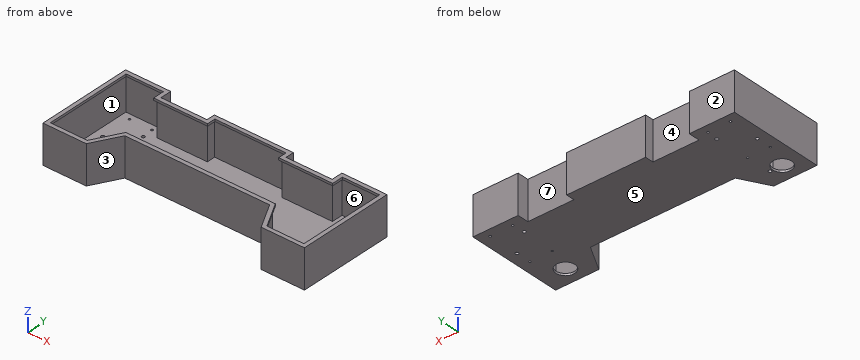
```python
from build123d import *

# Parameters (mm, degrees)
EXTRUDE_1_DEPTH         = 20.5
SCALE_1_SCALE           = 10
SHELL_1_T               = -11
EXTRUDE_2_DEPTH         = 12
HOLE_WIZARD_17_0_17_1_D = 17
M12X1_25_2_D            = 10.5
F_12_0MM_1_D            = 12
SKETCH_27_R             = 50
CUT_EXTRUDE_1_DEPTH     = 11


with BuildPart() as part:
    # 草图1 → 凸台-拉伸1 (new body)
    with BuildSketch(Plane.XY):
        Polygon((-61.070262854, 36.5), (-37.070262854, 36.5), (-37.070262854, 30.5), (-12.570262854, 30.5), (-12.570262854, 35), (29.429737146, 35), (29.429737146, 30.5), (53.929737146, 30.5), (53.929737146, 36.5), (77.929737146, 36.5), (77.929737146, -14.5), (54.929737146, -14.5), (46.929737146, 0), (-30.070262854, 0), (-38.070262854, -14.5), (-61.070262854, -14.5), align=None)
    extrude(amount=EXTRUDE_1_DEPTH)


with BuildPart() as part_1:
    # 缩放比例1: scaled about (8.429737146, 13.654642846, 10.25)
    add(part.part.scale(SCALE_1_SCALE).moved(Location((-75.867634314, -122.891785614, -92.25))))

    # 抽壳1
    shell_1_openings = [part_1.faces().sort_by_distance(p)[0] for p in [
        (8.429737147, 13.654642849, 112.75),
    ]]
    offset(amount=SHELL_1_T, openings=shell_1_openings, kind=Kind.INTERSECTION)

    # 草图12 → 凸台-拉伸2 (add)
    with BuildSketch(Plane.XY.offset(112.75)):
        Polygon((-675.570262854, 231.108214383), (-675.570262854, -256.891785617), (-463.064431597, -256.891785617), (-383.064431597, -111.891785617), (399.923905889, -111.891785617), (479.923905889, -256.891785617), (692.429737146, -256.891785617), (692.429737146, 231.108214383), (474.429737146, 231.108214383), (474.429737146, 171.108214383), (207.429737146, 171.108214383), (207.429737146, 216.108214383), (-190.570262854, 216.108214383), (-190.570262854, 171.108214383), (-457.570262854, 171.108214383), (-457.570262854, 231.108214383), align=None)
        Polygon((-665.570262854, 221.108214383), (-665.570262854, -246.891785617), (-468.968221364, -246.891785617), (-388.968221364, -101.891785617), (405.827695656, -101.891785617), (485.827695656, -246.891785617), (682.429737146, -246.891785617), (682.429737146, 221.108214383), (484.429737146, 221.108214383), (484.429737146, 161.108214383), (197.429737146, 161.108214383), (197.429737146, 206.108214383), (-180.570262854, 206.108214383), (-180.570262854, 161.108214383), (-467.570262854, 161.108214383), (-467.570262854, 221.108214383), align=None, mode=Mode.SUBTRACT)
    extrude(amount=-EXTRUDE_2_DEPTH)

    # Ø17.0 (17) 直径孔1 (through all)
    with Locations(Plane.XY.offset(-81.25)):
        with Locations((-505.570262854, 141.108214383), (-630.570262854, 36.108214383), (-515.570262854, -176.891785617), (647.429737146, 36.108214383), (522.429737146, 136.108214383), (532.429737146, -176.891785617)):
            Hole(HOLE_WIZARD_17_0_17_1_D / 2)

    # M12x1.25 螺纹孔2 (through all)
    with Locations(Plane.XY.offset(-81.25)):
        with Locations((-630.570262854, -43.891785617), (-510.570262854, -43.891785617), (527.429737146, -43.891785617), (647.429737146, -43.891785617)):
            Hole(M12X1_25_2_D / 2)

    # Ø12.0mm 暗销孔1 (through all)
    with Locations(Plane(origin=(-630.570262854, 201.108214383, -81.25), x_dir=(1, 0, 0), z_dir=(0, 0, 1))):
        with Locations((0, 0), (120, 0), (1158, 0), (1278, 0)):
            Hole(F_12_0MM_1_D / 2)

    # 草图27 → 切除-拉伸1 (cut)
    with BuildSketch(Plane.XY.offset(-81.25)):
        with Locations((572.429737146, -176.891785617)):
            Circle(SKETCH_27_R)
        with Locations((-579.570262855, -176.891785617)):
            Circle(SKETCH_27_R)
    extrude(amount=-CUT_EXTRUDE_1_DEPTH, mode=Mode.SUBTRACT)


solid = part_1.part
```
Source: CAD feature listing. Evaluate the final solid. Frame: model axes, mm. Face numbers are marked on the shaded views. A direction names the side the tool comes from. Coordinates: 2 decimals unless noted, no trailing zeros. Write each loop counter-clockwise with the first axis right and the second up, starting at its lowest first coordinate (ties: lowest second). Pieces come first, ordered by that corner, then holes. Notation, with made-up numbers: (64, 26) -> (113, 26) arc R28 ccw to (113, 51) -> close; hole circle Ø6 at (-29.75, 36). An arc over 180 degrees is marked (long way). Return JSON: item names as keys, results as strings. Group by question number.
1) Section query C-C, the plane y = -66. Return loops of the section in (x, z).
2) Section query B-B, the plane x = -292. Return loops of the section in (y, z), plus the area to 3 significant figures.
3) Mould query, pull axis Z, two halves, no side actions, for the marked faces 5, 6 and 7. Classes: +Z half, -Z half, draft (parallel to the pull), parting line (faces both ways), or undercut.
4) Set-up query: the marked faces 1, 2, 3 and 4. Return all of +Z, -Z, +X, -X, +Y, -Y with unobstructed straight access to the full face (end or side cutting, diameter ignored); none if empty.
5) Ray query, line 1 along X through (y, z) = (186, 27.5); line 2 along X through (y, z) = (27, 56.5); line 3 along Y through (x, z) = (197.5, 95.5). Return the intervals inside material, ascending.
6) Contact query for flat-ended pins moving along their axis: P1, Ø2, axis at x = -332, z = 69.5, coming from the +Y side; P2, Ø12, axis at x = 647.43, y = -43.89, coming from the +Z side; P3, Ø1, axis at x = -221.5, z = 73, coming from the -Y side. Output: stop coordinate, or through.
From the geometry:
{
 "1": {"outline": "(-686.57, -92.25) -> (703.43, -92.25) -> (703.43, 112.75) -> (682.43, 112.75) -> (682.43, 100.75) -> (692.43, 100.75) -> (692.43, -81.25) -> (-675.57, -81.25) -> (-675.57, 100.75) -> (-665.57, 100.75) -> (-665.57, 112.75) -> (-686.57, 112.75) -> close"},
 "2": {"outline": "(-122.89, -92.25) -> (182.11, -92.25) -> (182.11, 112.75) -> (161.11, 112.75) -> (161.11, 100.75) -> (171.11, 100.75) -> (171.11, -81.25) -> (-111.89, -81.25) -> (-111.89, 100.75) -> (-101.89, 100.75) -> (-101.89, 112.75) -> (-122.89, 112.75) -> close", "area": "7,860 mm²"},
 "3": {"face 5": "-Z half", "face 6": "undercut", "face 7": "draft"},
 "4": {"face 1": "none", "face 2": "+Z, -Z, +X, -X, +Y", "face 3": "+Z, -Z, -Y", "face 4": "+Z, -Z, +Y"},
 "5": {"line 1": "-686.57 to -675.57, -457.57 to -446.57, -201.57 to -190.57, 207.43 to 218.43, 463.43 to 474.43, 692.43 to 703.43", "line 2": "-686.57 to -675.57, 692.43 to 703.43", "line 3": "-122.89 to -111.89, 216.11 to 227.11"},
 "6": {"P1": "y = 182.11", "P2": "z = -81.25", "P3": "y = -122.89"}
}
